The listing builds one solid part. Answer for the finished solid, in the listing's coordinates (mm). A direction names the side the tool comes from. Give positions to 0.01 mm unless a question says otherwise; leave off trailing zeros. Loops run counter-clockwise (first coordinate to the right, second up) from the corner with the lowest first, then second, coordinate; pieces in that order, holes last. Notation, with made-up numbers: M 89,26 L 131,26 A10 cw 131,37 Z; hole C 44.25,20 d9. An arc over 180 degrees is marked long. Use one line per item in the form item = value. Start each with the question number.
1. The part is cut by section B-B (z = 3.75). Give the number of separate pieces and of enclosed holes in the cut face, and give its area (3 significant figures).
2. Each of these flat-tipped pins is pushed along its axis until it touches: pin 1 Ø2 at (y, z) = (6, 3) entering from +X; pin 2 Ø2 at (x, y) = (-39, 20.5) entering from -Z; pin 3 Ø4 at (x, y) = (9.5, 4.5) entering from +Z; pin 4 Ø2 at (x, z) = (-37, 4) entering from -Y. Where does it stop, or does it pass through?
3. The part is cut by section A-A (x = -21.2). Write down the section's boundary in (y, z), and give its area (3 significant figures).
4. The part is cut by section C-C (x = 28.7). Write down the section's boundary in (y, z).
5. The mould has two halves that part along Y. Classify faces 4 (the face through (-33.2, 7, 4)), 5 (the face through (-29, 3, 3)), 6 (the face through (-30.5, 13.48, 6.19)), 7 (the face through (-6, 2.5, 4)): released by +Y, released by -Y, zero draft, split by the parting line, or undercut.
6. For faces 1 (the face through (27.373, 14.617, 6.192)), 2 (the face through (25.7, 13, 4)), 3 (the face through (36, 9.7, 4)), determine the directions among +Z, -Z, +X, -X, +Y, -Y from which every point of the face is accessible in a straight line to the end or side of a thin tool.
7. Straight lines are drawn through the part: line 1 (Y direction, x = -39, z = 0.85); line 2 (X direction, y = 6, z = 3.5); line 3 (X direction, y = 15.5, z = 3.5). For each, find the intervals that lie inside material, in ascending order. Write a range as from..to.
8. The part is cut by section D-D (y = -5.5). Write down the section's boundary in (x, z).
from build123d import *

# Parameters (mm, degrees)
SKETCH1_W           = 85
SKETCH1_H           = 48
BOSS_EXTRUDE1_DEPTH = 1.6
SKETCH2_R           = 1.25
CUT_EXTRUDE1_DEPTH  = 5
FILLET1_R           = 3
SKETCH_1_W          = 6
SKETCH_1_H          = 6
EXTRUDE_1_DEPTH     = 4
SKETCH_2_W          = 6
SKETCH_2_H          = 6
EXTRUDE_2_DEPTH     = 4
SKETCH_3_R          = 1.8
EXTRUDE_3_DEPTH     = 1.2
FILLET_2_R          = 0.6


with BuildPart() as part:
    # Sketch1 → Boss-Extrude1 (new body)
    with BuildSketch(Plane.XY):
        Rectangle(SKETCH1_W, SKETCH1_H)
    extrude(amount=BOSS_EXTRUDE1_DEPTH)

    # Sketch2 → Cut-Extrude1 (cut)
    with BuildSketch(Plane.XY.offset(1.6)):
        with Locations((-39, 20.5)):
            Circle(SKETCH2_R)
        with Locations((39, 20.5)):
            Circle(SKETCH2_R)
        with Locations((39, -20.5)):
            Circle(SKETCH2_R)
        with Locations((-39, -20.5)):
            Circle(SKETCH2_R)
    extrude(amount=-CUT_EXTRUDE1_DEPTH, mode=Mode.SUBTRACT)

    # Fillet1
    fillet1_edges = [part.edges().sort_by_distance(p)[0] for p in [
        (-42.5, 24, 0.8),
        (42.5, 24, 0.8),
        (42.5, -24, 0.8),
        (-42.5, -24, 0.8),
    ]]
    fillet(fillet1_edges, radius=FILLET1_R)

    # 草图1 → 凸台-拉伸1 (add)
    with BuildSketch(Plane.XY.offset(1.6)):
        with Locations((-28.7, 13.4)):
            Rectangle(SKETCH_1_W, SKETCH_1_H)
        with Locations((-28.7, 0)):
            Rectangle(SKETCH_1_W, SKETCH_1_H)
        with Locations((-36.2, 6.7)):
            Rectangle(SKETCH_1_W, SKETCH_1_H)
        with Locations((-21.2, 6.7)):
            Rectangle(SKETCH_1_W, SKETCH_1_H)
    extrude_1 = extrude(amount=EXTRUDE_1_DEPTH)

    # 镜向1: 凸台-拉伸1 across plane
    add(extrude_1.mirror(Plane(origin=(0, 0, 0), x_dir=(0, 0, 1), z_dir=(1, 0, 0))))

    # 草图2 → 凸台-拉伸2 (add)
    with BuildSketch(Plane.XY.offset(1.6)):
        with Locations((-5.5, -0.5)):
            Rectangle(SKETCH_2_W, SKETCH_2_H)
        with Locations((5.5, -0.5)):
            Rectangle(SKETCH_2_W, SKETCH_2_H)
    extrude(amount=EXTRUDE_2_DEPTH)

    # 草图3 → 凸台-拉伸3 (add)
    with BuildSketch(Plane.XY.offset(5.6)):
        with Locations((-36.2, 6.7)):
            Circle(SKETCH_3_R)
        with Locations((-28.7, 13.4)):
            Circle(SKETCH_3_R)
        with Locations((-21.2, 6.7)):
            Circle(SKETCH_3_R)
        with Locations((-28.7, 0)):
            Circle(SKETCH_3_R)
        with Locations((-5.5, -0.5)):
            Circle(SKETCH_3_R)
        with Locations((5.5, -0.5)):
            Circle(SKETCH_3_R)
        with Locations((21.2, 6.7)):
            Circle(SKETCH_3_R)
        with Locations((28.7, 0)):
            Circle(SKETCH_3_R)
        with Locations((36.2, 6.7)):
            Circle(SKETCH_3_R)
        with Locations((28.7, 13.4)):
            Circle(SKETCH_3_R)
    extrude(amount=EXTRUDE_3_DEPTH)

    # 圆角2
    fillet_2_edges = [part.edges().sort_by_distance(p)[0] for p in [
        (25.7, 3, 3.6),
        (25.7, -3, 3.6),
        (31.7, -3, 3.6),
        (31.7, 3, 3.6),
        (39.2, 9.7, 3.6),
        (39.2, 3.7, 3.6),
        (33.2, 3.7, 3.6),
        (33.2, 9.7, 3.6),
        (31.7, 10.4, 3.6),
        (31.7, 16.4, 3.6),
        (25.7, 16.4, 3.6),
        (25.7, 10.4, 3.6),
        (18.2, 3.7, 3.6),
        (18.2, 9.7, 3.6),
        (24.2, 3.7, 3.6),
        (24.2, 9.7, 3.6),
        (8.5, 2.5, 3.6),
        (2.5, 2.5, 3.6),
        (2.5, -3.5, 3.6),
        (8.5, -3.5, 3.6),
        (-2.5, -3.5, 3.6),
        (-8.5, -3.5, 3.6),
        (-8.5, 2.5, 3.6),
        (-2.5, 2.5, 3.6),
        (-24.2, 9.7, 3.6),
        (-18.2, 3.7, 3.6),
        (-18.2, 9.7, 3.6),
        (-24.2, 3.7, 3.6),
        (-31.7, 3, 3.6),
        (-25.7, 3, 3.6),
        (-28.7, 3, 5.6),
        (-25.7, -3, 3.6),
        (-31.7, -3, 3.6),
        (-31.7, 16.4, 3.6),
        (-25.7, 16.4, 3.6),
        (-25.7, 10.4, 3.6),
        (-31.7, 10.4, 3.6),
        (-33.2, 9.7, 3.6),
        (-33.2, 3.7, 3.6),
        (-39.2, 3.7, 3.6),
        (-39.2, 9.7, 3.6),
    ]]
    fillet(fillet_2_edges, radius=FILLET_2_R)


solid = part.part
Derived:
q1.separate_pieces = 10
q1.enclosed_holes = 0
q1.area = 357 mm2
q2.pin_1 = 39.2
q2.pin_2 = through
q2.pin_3 = 1.6
q2.pin_4 = 3.7
q3.outline = M -24,0 L 24,0 L 24,1.6 L 9.7,1.6 L 9.7,5.6 L 8.5,5.6 L 8.5,6.8 L 4.9,6.8 L 4.9,5.6 L 3.7,5.6 L 3.7,1.6 L -24,1.6 Z
q3.area = 105 mm2
q4.outline = M -24,0 L 24,0 L 24,1.6 L 16.4,1.6 L 16.4,5.6 L 15.2,5.6 L 15.2,6.8 L 11.6,6.8 L 11.6,5.6 L 10.4,5.6 L 10.4,1.6 L 3,1.6 L 3,5.6 L 1.8,5.6 L 1.8,6.8 L -1.8,6.8 L -1.8,5.6 L -3,5.6 L -3,1.6 L -24,1.6 Z
q5.face_4 = zero draft
q5.face_5 = undercut
q5.face_6 = undercut
q5.face_7 = released by +Y
q6.face_1 = +Z
q6.face_2 = +Z, +Y, -Y
q6.face_3 = +Z, +X, -X, +Y
q7.line_1 = -24..-21.75, -19.25..19.25, 21.75..24
q7.line_2 = -39.2..-33.2, -24.2..-18.2, 18.2..24.2, 33.2..39.2
q7.line_3 = -31.7..-25.7, 25.7..31.7
q8.outline = M -42.5,0 L 42.5,0 L 42.5,1.6 L -42.5,1.6 Z
